Source: three-view drawing plus pictorial views. Frame: mm from the lowest corner of the part. A direction names the side the tool comes from. Round coordinates to 2 decimals unless told otherwise and drop trailing zeros. Loops run counter-clockwise (first coordinate to the right, second up) from the corner with the lowest first, then second, coordinate; pieces in that order, holes last. Notation, with made-up numbers: (-11, 21) -> (34, 21) arc R7 cw to (34, 30) -> close; hole circle Ø1 at (50, 5.5). An arc over 180 degrees is marked (long way). Return JSON: item names as keys, results as strings. Group by question number.
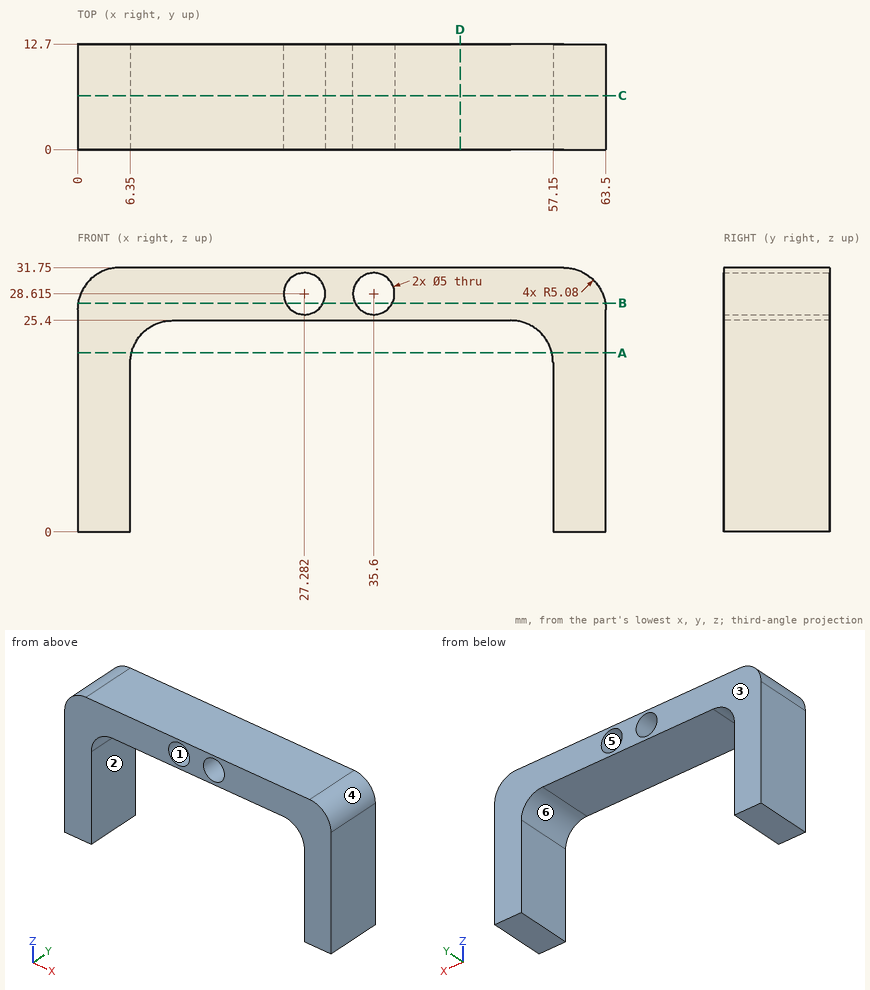
(1) Pin query (flat end, axial travel): pin 1 (3 mm diameter, centred on x = 27.28, z = 28.62, fed in from -Y). Return the tip coordinate at first contact, or that it passes through.
(2) Cut plane A-A (z = 21.5). Return loops of the section in (x, y), and give its area (3 significant figures).
(3) Cut plane D-D (x = 46). Return loops of the section in (y, z).
(4) Set-up query: the marked faces 1 and 2. Return all of +Z, -Z, +X, -X, +Y, -Y with unobstructed straight access to the full face (end or side cutting, diameter ignored); none if empty.
(5) Mould query, pull axis Z, two halves, no side actions, for the marked faces 3, 4, 5 and 6. Classes: released by +Z, released by -Z, zero draft, split by the parting line, or undercut.
(6) Ray query, line 1 (X direction, y = 3, z = 18); line 2 (X direction, y = 8.75, z = 27.5) (1 decimal). Return the intervals inside material, ascending.
(7) Cut plane C-C (y = 6.5). Count the separate pieces of the cut face and the enclosed holes in it.
(8) Cut plane B-B (z = 27.5). Return loops of the section in (x, y), and give its area (3 significant figures).
Answers follow:
{
 "1": {"pin 1": "through"},
 "2": {"outline": "(0, 0) -> (6.49, 0) -> (6.49, 12.7) -> (0, 12.7) -> close; (57.01, 0) -> (63.5, 0) -> (63.5, 12.7) -> (57.01, 12.7) -> close", "area": "165 mm^2"},
 "3": {"outline": "(0, 25.4) -> (12.7, 25.4) -> (12.7, 31.75) -> (0, 31.75) -> close"},
 "4": {"face 1": "+Y, -Y", "face 2": "-Z, +Y, -Y"},
 "5": {"face 3": "zero draft", "face 4": "released by +Z", "face 5": "undercut", "face 6": "released by -Z"},
 "6": {"line 1": "0 to 6.35, 57.15 to 63.5", "line 2": "0.1 to 25, 29.5 to 33.4, 37.8 to 63.4"},
 "7": {"separate pieces": "1", "enclosed holes": "2"},
 "8": {"outline": "(0.07, 0) -> (25.04, 0) -> (25.04, 12.7) -> (0.07, 12.7) -> close; (29.52, 0) -> (33.36, 0) -> (33.36, 12.7) -> (29.52, 12.7) -> close; (37.84, 0) -> (63.43, 0) -> (63.43, 12.7) -> (37.84, 12.7) -> close", "area": "691 mm^2"}
}
